The model under review builds one solid part; all positions refer to its coordinate system, in mm. A direction names the side the tool comes from. Coordinates: 2 decimals unless noted, no trailing zeros. Order: outer loops, then holes, each group sorted by start corner. A loop starts at its lowest first (then second) coordinate and runs counter-clockwise, first axis right, second up. Notation, with made-up numbers: (20.5, 71) - (60.5, 71) arc R30 cw to (60.5, 109) - close; hole circle Ø3 at (30, 45.5). An arc over 180 degrees is marked (long way). Answer in a Markdown table with one row per item.
```python
from build123d import *

# Parameters (mm, degrees)
F1_DEPTH = 37.5
F3_DEPTH = 25


# Not quite as in the source:
# - ends of sketch curves that miss each other by under 0.0002 mm in the source are joined


with BuildPart() as f1:
    # F0 (on Top) → F1 (new body)
    with BuildSketch(Plane.XY):
        with BuildLine():
            Line((-87.240451, 4.779809), (-87.240451, -5.411983))
            Line((-87.240451, -5.411983), (-87.240451, -7.720191))
            Line((-87.240451, -7.720191), (-87.240451, -17.023544))
            Line((-87.240451, -17.023544), (-87.240451, -20.220191))
            Line((-87.240451, -20.220191), (-87.240451, -23.220191))
            Line((-87.240451, -23.220191), (-86.240451, -23.220191))
            Line((-86.240451, -23.220191), (-84.740451, -21.720191))
            Line((-84.740451, -21.720191), (-81.394629, -21.720191))
            ThreePointArc((-81.394629, -21.720191), (-81.2725220613, -21.7617930975), (-81.2012141703, -21.8692920448))
            Line((-81.2012141703, -21.8692920448), (-80.747036, -23.595168))
            ThreePointArc((-80.747036, -23.595168), (-80.7421040626, -23.6204048929), (-80.740451, -23.646066))
            Line((-80.740451, -23.646066), (-80.740451, -25.020191))
            ThreePointArc((-80.740451, -25.020191), (-80.6818723562, -25.1616123562), (-80.540451, -25.220191))
            Line((-80.540451, -25.220191), (-79.940451, -25.220191))
            ThreePointArc((-79.940451, -25.220191), (-79.7990296438, -25.1616123562), (-79.740451, -25.020191))
            Line((-79.740451, -25.020191), (-79.740451, -21.220191))
            ThreePointArc((-79.740451, -21.220191), (-80.0333442188, -20.5130842188), (-80.740451, -20.220191))
            Line((-80.740451, -20.220191), (-85.740451, -20.220191))
            Line((-85.740451, -20.220191), (-85.740451, -7.720191))
            Line((-85.740451, -7.720191), (-85.740451, 4.779809))
            Line((-85.740451, 4.779809), (-80.740451, 4.779809))
            ThreePointArc((-80.740451, 4.779809), (-80.0333442188, 5.0727022188), (-79.740451, 5.779809))
            Line((-79.740451, 5.779809), (-79.740451, 9.579809))
            ThreePointArc((-79.740451, 9.579809), (-79.7990296438, 9.7212303562), (-79.940451, 9.779809))
            Line((-79.940451, 9.779809), (-80.540451, 9.779809))
            ThreePointArc((-80.540451, 9.779809), (-80.6818723562, 9.7212303562), (-80.740451, 9.579809))
            Line((-80.740451, 9.579809), (-80.740451, 8.205684))
            ThreePointArc((-80.740451, 8.205684), (-80.7421040626, 8.1800228929), (-80.7470359242, 8.15478598))
            Line((-80.7470359242, 8.15478598), (-81.201214, 6.42891))
            ThreePointArc((-81.201214, 6.42891), (-81.2725220613, 6.3214110975), (-81.394629, 6.279809))
            Line((-81.394629, 6.279809), (-84.740451, 6.279809))
            Line((-84.740451, 6.279809), (-86.240451, 7.779809))
            Line((-86.240451, 7.779809), (-87.240451, 7.779809))
            Line((-87.240451, 7.779809), (-87.240451, 4.779809))
        make_face()
    extrude(amount=F1_DEPTH)

    # F2 (on face) → F3 (cut)
    with BuildSketch(Plane.YZ.offset(-85.740451)):
        with BuildLine():
            ThreePointArc((-10.470191, 23.75), (-7.720191, 21), (-4.970191, 23.75))
            Line((-4.970191, 23.75), (-4.970191, 26.25))
            ThreePointArc((-4.970191, 26.25), (-7.720191, 29), (-10.470191, 26.25))
            Line((-10.470191, 26.25), (-10.470191, 23.75))
        make_face()
        with BuildLine():
            Line((-4.970191, 11.25), (-4.970191, 13.75))
            ThreePointArc((-4.970191, 13.75), (-7.720191, 16.5), (-10.470191, 13.75))
            Line((-10.470191, 13.75), (-10.470191, 11.25))
            ThreePointArc((-10.470191, 11.25), (-7.720191, 8.5), (-4.970191, 11.25))
        make_face()
        with BuildLine():
            Line((-4.970191, -1.25), (-4.970191, 1.25))
            ThreePointArc((-4.970191, 1.25), (-7.720191, 4), (-10.470191, 1.25))
            Line((-10.470191, 1.25), (-10.470191, -1.25))
            ThreePointArc((-10.470191, -1.25), (-7.720191, -4), (-4.970191, -1.25))
        make_face()
        with BuildLine():
            Line((-4.970191, 36.25), (-4.970191, 38.75))
            ThreePointArc((-4.970191, 38.75), (-7.720191, 41.5), (-10.470191, 38.75))
            Line((-10.470191, 38.75), (-10.470191, 36.25))
            ThreePointArc((-10.470191, 36.25), (-7.720191, 33.5), (-4.970191, 36.25))
        make_face()
    extrude(amount=-F3_DEPTH, mode=Mode.SUBTRACT)


solid = f1.part
```
Item 1: We need section B-B, the plane y = -7. Write out the cut boundary in (x, z), then the cut area to 3 significant figures.
Check values:
| item | result |
|---|---|
| outline | (-87.24, 3.9) - (-85.74, 3.9) - (-85.74, 8.6) - (-87.24, 8.6) - close; (-87.24, 16.4) - (-85.74, 16.4) - (-85.74, 21.1) - (-87.24, 21.1) - close; (-87.24, 28.9) - (-85.74, 28.9) - (-85.74, 33.6) - (-87.24, 33.6) - close |
| area | 21.1 mm^2 |
Item 2: To check wall thickness, follow line 1 (Y direction, x = -81.5, z = 2.5); line 2 (X direction, y = -11, z = 19.5); line 3 (Y direction, x = -80, z = 30). State the ranges of each line that lie inside material, in increasing order. Write a range as from..to.
Check values:
| item | result |
|---|---|
| line 1 | -21.72..-20.22, 4.78..6.28 |
| line 2 | -87.24..-85.74 |
| line 3 | -25.22..-20.55, 5.11..9.78 |
Item 3: We need section D-D, the plane z = 5. Write out the cut boundary in (x, y).
Check values:
| item | result |
|---|---|
| outline | (-87.24, -23.22) - (-86.24, -23.22) - (-84.74, -21.72) - (-81.39, -21.72) arc R0.2 cw to (-81.2, -21.87) - (-80.75, -23.6) arc R0.2 cw to (-80.74, -23.65) - (-80.74, -25.02) arc R0.2 ccw to (-80.54, -25.22) - (-79.94, -25.22) arc R0.2 ccw to (-79.74, -25.02) - (-79.74, -21.22) arc R1 ccw to (-80.74, -20.22) - (-85.74, -20.22) - (-85.74, 4.78) - (-80.74, 4.78) arc R1 ccw to (-79.74, 5.78) - (-79.74, 9.58) arc R0.2 ccw to (-79.94, 9.78) - (-80.54, 9.78) arc R0.2 ccw to (-80.74, 9.58) - (-80.74, 8.21) arc R0.2 cw to (-80.75, 8.15) - (-81.2, 6.43) arc R0.2 cw to (-81.39, 6.28) - (-84.74, 6.28) - (-86.24, 7.78) - (-87.24, 7.78) - close |
Item 4: Clearance check with flat-ended pins moving along their axes: pin 1 Ø1.1 at (x, z) = (-86.5, 18.5) entering from +Y; pin 2 Ø1.4 at (x, z) = (-86.5, 0.5) entering from -Y; pin 3 Ø1.5 at (x, y) = (-86, -8) entering from -Z. State where each tip first meets the part, or that it passes through.
Check values:
| item | result |
|---|---|
| pin 1 | y = 7.78 |
| pin 2 | y = -23.22 |
| pin 3 | z = 3.8 |
Item 5: Tool access review of faces 1 (the face through (-80.74, 9, 18)), 2 (the face through (-87, -23.22, 18)), 3 (the face through (-85.5, -22.48, 18.49)): name each direction out of +Z, -Z, +X, -X, +Y, -Y from which nothing blocks a thin tool from reaching the whole face with its end or side.
Check values:
| item | result |
|---|---|
| face 1 | +Z, -Z, -X, +Y |
| face 2 | +Z, -Z, -X, -Y |
| face 3 | +Z, -Z, -Y |
Item 6: We need section A-A, the plane x = -83.25. Write out the cut boundary in (y, z), then the cut area to 4 significant figures.
Check values:
| item | result |
|---|---|
| outline | (-21.72, 0) - (-20.22, 0) - (-20.22, 37.5) - (-21.72, 37.5) - close; (4.78, 0) - (6.28, 0) - (6.28, 37.5) - (4.78, 37.5) - close |
| area | 112.5 mm^2 |
Item 7: Mouldability with a two-part tool opening along Z and no side actions: class faces 4 (the face through (-80.74, -24, 18)), 5 (the face through (-86.5, -7.7, 16.5)), 6 (the face through (-85, -21, 37.5)), 7 (the face through (-86.5, -7.7, 4)) as +Z half, -Z half, draft (parallel to the pull), parting line (faces both ways), or undercut.
Check values:
| item | result |
|---|---|
| face 4 | draft |
| face 5 | undercut |
| face 6 | +Z half |
| face 7 | -Z half |
